Build history of the part. All positions in model axes, mm. A direction names the side the tool comes from. Coordinates: 2 decimals unless noted, no trailing zeros. Order: outer loops, then holes, each group sorted by start corner. A loop starts at its lowest first (then second) coordinate and runs counter-clockwise, first axis right, second up. Notation, with made-up numbers: (32.5, -6) -> (61.5, -6) arc R12 ccw to (61.5, 1) -> close; hole circle Ø6 at (18.25, 89.5). An arc over 180 degrees is marked (long way). Write each question's results on one line, items separated by ' | '.
from build123d import *

# Parameters (mm, degrees)
ESBO_O1_R                  = 15
ESBO_O1_W                  = 12.25
ESBO_O1_H                  = 12.25
RESSALTO_EXTRUS_O1_DEPTH   = 10
CORTE_EXTRUS_O1_DEPTH      = 24
CORTE_EXTRUS_O1_DEPTH_BACK = 24
ESBO_O2_R                  = 2.35


with BuildPart() as part:
    # Esboço1 → Ressalto-extrusão1 (new body)
    with BuildSketch(Plane.XY):
        Circle(ESBO_O1_R)
        Rectangle(ESBO_O1_W, ESBO_O1_H, mode=Mode.SUBTRACT)
    extrude(amount=RESSALTO_EXTRUS_O1_DEPTH)

    # Esboço2 → Corte-extrusão1 (cut, two sides: drawn at the far end of the back side and taken through both)
    with BuildSketch(Plane(origin=(0, 0, 0), x_dir=(1, 0, 0), z_dir=(0, 1, 0)).offset(-CORTE_EXTRUS_O1_DEPTH_BACK)):
        with Locations(Location((0, -5, 0), (0, 0, 90))):
            Circle(ESBO_O2_R)
    extrude(amount=CORTE_EXTRUS_O1_DEPTH + CORTE_EXTRUS_O1_DEPTH_BACK, mode=Mode.SUBTRACT)


solid = part.part
Item 1: Drill centre lines: line 1 (X direction, y = -0.5, z = 5.75) (3 decimals); line 2 (X direction, y = -11.5, z = 5). Where is each one in solid material? Low to high. Write a range as from..to.
Answer:
line 1: x = -14.992..-6.125, 6.125..14.992 | line 2: x = -9.63..-2.35, 2.35..9.63
Item 2: Pull direction Y, two halves, no side cores. Call faces 3 (the flat face through (6.125, 0, 5)), 4 (the flat face through (1.3, 6.125, 2.7)), 5 (the cylindrical face through (-3.252, -14.643, 4.93)), 6 (the flat face through (6.5, 0.2, 0)): released by +Y, released by -Y, zero draft, split by the parting line, or undercut.
Answer:
face 3: undercut | face 4: undercut | face 5: split by the parting line | face 6: zero draft
Item 3: Tool access for faces 1 (the flat face through (-6.125, 0, 5)), 2 (the cylindrical face through (-0.71, 10.5, 2.76)): list every direction of +Z, -Z, +X, -X, +Y, -Y with a clear straight run to the whole face (end or side of a thin tool).
Answer:
face 1: +Z, -Z | face 2: +Y, -Y
Item 4: Slice it at A-A, the plane y = 0. List the corners of the cut face in (x, z) (3 decimals).
Answer:
outline: (-15, 0) -> (-6.125, 0) -> (-6.125, 10) -> (-15, 10) -> close; (6.125, 0) -> (15, 0) -> (15, 10) -> (6.125, 10) -> close
Item 5: Slice it at B-B, the plane z = 8.5. List the corners of the cut face in (x, y) (3 decimals).
Answer:
outline: circle Ø30 at (0, 0); hole (-6.125, -6.125) -> (6.125, -6.125) -> (6.125, 6.125) -> (-6.125, 6.125) -> close
Item 6: Slice it at C-C, the plane x = 0. List the corners of the cut face in (y, z) (3 decimals), and give its area (3 significant figures).
Answer:
outline: (-15, 0) -> (-6.125, 0) -> (-6.125, 2.65) -> (-15, 2.65) -> close; (-15, 7.35) -> (-6.125, 7.35) -> (-6.125, 10) -> (-15, 10) -> close; (6.125, 0) -> (15, 0) -> (15, 2.65) -> (6.125, 2.65) -> close; (6.125, 7.35) -> (15, 7.35) -> (15, 10) -> (6.125, 10) -> close | area: 94.1 mm^2
Item 7: Pin check, flat tips, straight feed: pin 1 (1 mm diameter, centred on x = 1, z = 1, fed in from -Y); pin 2 (1.5 mm diameter, centred on y = -4, z = 4.5, fed in from +X); pin 3 (5 mm diameter, centred on y = -3, z = 3.5, fed in from +X). Stop position of each tip, or through.
Answer:
pin 1: stops at y = -14.99 | pin 2: stops at x = 14.64 | pin 3: stops at x = 14.99
Item 8: Slice it at D-D, the plane z = 4.25. List the corners of the cut face in (x, y) (3 decimals).
Answer:
outline: (-6.125, -6.125) -> (-6.125, 6.125) -> (-2.227, 6.125) -> (-2.227, 14.834) arc R15 ccw to (-2.227, -14.834) -> (-2.227, -6.125) -> close; (2.227, -14.834) arc R15 ccw to (2.227, 14.834) -> (2.227, 6.125) -> (6.125, 6.125) -> (6.125, -6.125) -> (2.227, -6.125) -> close
